Could you check a few things on this model? Use its own coordinates, in mm. Face numbers are marked on the shaded views. A direction names the side the tool comes from. Round coordinates to 2 decimals unless told otherwise and drop trailing zeros. Loops run counter-clockwise (first coordinate to the right, second up) from the corner with the lowest first, then second, coordinate; pieces in that order, holes last.
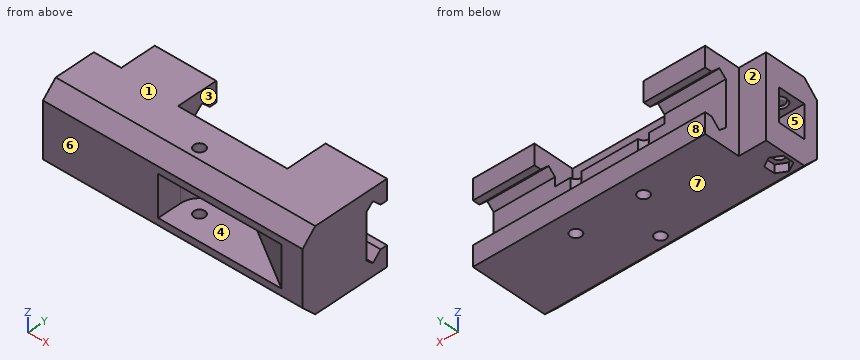
from build123d import *

# Parameters (mm, degrees)
SKETCH_1_W               = 30
SKETCH_1_H               = 20
SKETCH_1_W_2             = 12
SKETCH_1_H_2             = 10
EXTRUDE_1_DEPTH          = 10
CUT_EXTRUDE_1_DEPTH      = 3
SKETCH_4_R               = 1.95
CUT_EXTRUDE_2_DEPTH      = 30
SKETCH_8_R               = 2.8
SKETCH_8_R_2             = 2.2
CUT_EXTRUDE_3_DEPTH      = 5
FILLET_1_R               = 1
SKETCH_12_W              = 85
SKETCH_12_H              = 33.2
EXTRUDE_3_DEPTH          = 15
CUT_EXTRUDE_4_DEPTH      = 100
CHAMFER_1_SIZE           = 5
CUT_EXTRUDE_5_DEPTH      = 99.935534567
CUT_EXTRUDE_5_DEPTH_BACK = 99.935534567
SKETCH_14_R              = 2
CUT_EXTRUDE_6_DEPTH      = 7.5
CUT_EXTRUDE_7_DEPTH      = 99.935534567
CUT_EXTRUDE_7_DEPTH_BACK = 99.935534567
SKETCH_16_R              = 2
SKETCH_17_W              = 40
SKETCH_17_H              = 15
CUT_EXTRUDE_8_DEPTH      = 10


with BuildPart() as part:
    # 스케치1 → 보스-돌출1 (new body)
    with BuildSketch(Plane(origin=(0, 0, 0), x_dir=(0, 0, -1), z_dir=(1, 0, 0))):
        Rectangle(SKETCH_1_W, SKETCH_1_H)
        Rectangle(SKETCH_1_W_2, SKETCH_1_H_2, mode=Mode.SUBTRACT)
    extrude(amount=EXTRUDE_1_DEPTH)

    # 스케치2 → 컷-돌출1 (cut)
    with BuildSketch(Plane(origin=(0, 0, -15), x_dir=(-1, 0, 0), z_dir=(0, 0, -1))):
        Polygon((-1.175, -2.006292185), (-1.175, 2.006292185), (-4.65, 4.012584371), (-8.125, 2.006292185), (-8.125, -2.006292185), (-4.65, -4.012584371), align=None)
    extrude(amount=-CUT_EXTRUDE_1_DEPTH, mode=Mode.SUBTRACT)

    # 스케치4 → 컷-돌출2 (cut)
    with BuildSketch(Plane.XY):
        with Locations(Location((4.65, 0, 0), (0, 0, 270))):
            Circle(SKETCH_4_R)
    extrude(amount=-CUT_EXTRUDE_2_DEPTH, mode=Mode.SUBTRACT)

    # 스케치8 → 컷-돌출3 (cut)
    with BuildSketch(Plane(origin=(0, 0, 6), x_dir=(-1, 0, 0), z_dir=(0, 0, -1))):
        with Locations(Location((-4.65, 0, 0), (0, 0, 90))):
            Circle(SKETCH_8_R)
        with Locations(Location((-4.65, 0, 0), (0, 0, 90))):
            Circle(SKETCH_8_R_2, mode=Mode.SUBTRACT)
    extrude(amount=-CUT_EXTRUDE_3_DEPTH, mode=Mode.SUBTRACT)

    # 필렛1
    fillet_1_edges = [part.edges().sort_by_distance(p)[0] for p in [
        (4.65, -2.2, 6),
    ]]
    fillet(fillet_1_edges, radius=FILLET_1_R)

    # 스케치12 → 보스-돌출3 (add, symmetric)
    with BuildSketch(Plane.XY):
        with Locations((52.5, 6.6)):
            Rectangle(SKETCH_12_W, SKETCH_12_H)
    extrude(amount=EXTRUDE_3_DEPTH, both=True)

    # 스케치13 → 컷-돌출4 (cut, symmetric)
    with BuildSketch(Plane(origin=(0, 0, 0), x_dir=(0, 0, -1), z_dir=(1, 0, 0))):
        Polygon((7.6, 23.2), (-7.6, 23.2), (-7.6, 20.7), (-10.5, 17.7), (-10.5, 17.6), (-8.25, 15.1), (8.25, 15.1), (10.5, 17.6), (10.5, 17.7), (7.6, 20.7), align=None)
    extrude(amount=CUT_EXTRUDE_4_DEPTH, both=True, mode=Mode.SUBTRACT)

    # 모따기1
    chamfer_1_edges = [part.edges().sort_by_distance(p)[0] for p in [
        (47.5, -10, -15),
        (47.5, -10, 15),
    ]]
    chamfer(chamfer_1_edges, length=CHAMFER_1_SIZE)

    # 스케치14 → 컷-돌출5 (cut, two sides: drawn at the far end of the back side and taken through both)
    with BuildSketch(Plane.XY.offset(-CUT_EXTRUDE_5_DEPTH_BACK)):
        with Locations(Location((40.1, 15.1, 0), (0, 0, 90))):
            Circle(SKETCH_14_R)
        with Locations(Location((64.9, 15.1, 0), (0, 0, 90))):
            Circle(SKETCH_14_R)
    extrude(amount=CUT_EXTRUDE_5_DEPTH + CUT_EXTRUDE_5_DEPTH_BACK, mode=Mode.SUBTRACT)

    # 스케치15 → 컷-돌출6 (cut, symmetric)
    with BuildSketch(Plane.XY):
        with BuildLine():
            Line((62.713186115, 5.72501597), (49.092705045, 5.72501597))
            ThreePointArc((49.092705045, 5.72501597), (44.199467341, 3.698170549), (42.17262192, -1.195067155))
            Line((42.17262192, -1.195067155), (42.17262192, -12.628733774))
            Line((42.17262192, -12.628733774), (87.317926114, -12.628733774))
            Line((87.317926114, -12.628733774), (87.317926114, -10))
            Line((87.317926114, -10), (62.713186115, 5.72501597))
        make_face()
    extrude(amount=CUT_EXTRUDE_6_DEPTH, both=True, mode=Mode.SUBTRACT)

    # 스케치16 → 컷-돌출7 (cut, two sides: drawn at the far end of the back side and taken through both)
    with BuildSketch(Plane.XY.offset(-CUT_EXTRUDE_7_DEPTH_BACK)):
        with Locations((49.092705045, -1.195067155)):
            Circle(SKETCH_16_R)
    extrude(amount=CUT_EXTRUDE_7_DEPTH + CUT_EXTRUDE_7_DEPTH_BACK, mode=Mode.SUBTRACT)

    # 스케치17 → 컷-돌출8 (cut)
    with BuildSketch(Plane.XY.offset(15)):
        with Locations((52.5, 15.7)):
            Rectangle(SKETCH_17_W, SKETCH_17_H)
    extrude(amount=-CUT_EXTRUDE_8_DEPTH, mode=Mode.SUBTRACT)


solid = part.part
Item 1: We'd pull the mould along Y, two halves only. Please class the marked faces 5, 6, 7 and 8: released by +Y, released by -Y, zero draft, split by the parting line, or undercut.
Results list:
face 5: undercut
face 6: released by -Y
face 7: zero draft
face 8: released by +Y
Item 2: If we section it at D-D, the plane z = 3.5: Please give me the cut outline in (x, y).
Results list:
outline: (0, -10) - (42.17, -10) - (42.17, -1.2) arc R6.92 cw to (49.09, 5.73) - (62.71, 5.73) - (87.32, -10) - (95, -10) - (95, 15.1) - (66.9, 15.1) arc R2 cw to (62.9, 15.1) - (42.1, 15.1) arc R2 cw to (38.1, 15.1) - (10, 15.1) - (10, 10) - (0, 10) - (0, 5) - (10, 5) - (10, -5) - (0, -5) - close
Item 3: If we section it at B-B, the plane y = 11.5: Please give me the cut outline in (x, z), then the cut area to 3 significant figures.
Results list:
outline: (10, -15) - (95, -15) - (95, 15) - (72.5, 15) - (72.5, 5) - (32.5, 5) - (32.5, 15) - (10, 15) - close
area: 2,150 mm2
Item 4: If we section it at C-C, the plane x = 19.5: Please give me the cut outline in (y, z).
Results list:
outline: (-10, -10) - (-5, -15) - (23.2, -15) - (23.2, -7.6) - (20.7, -7.6) - (17.7, -10.5) - (17.6, -10.5) - (15.1, -8.25) - (15.1, 8.25) - (17.6, 10.5) - (17.7, 10.5) - (20.7, 7.6) - (23.2, 7.6) - (23.2, 15) - (-5, 15) - (-10, 10) - close
Item 5: If we section it at A-A, the plane x = 40.1: Please give me the cut outline in (y, z).
Results list:
outline: (-10, -10) - (-5, -15) - (13.1, -15) - (13.1, 5) - (8.2, 5) - (8.2, 15) - (-5, 15) - (-10, 10) - close; (17.1, -15) - (23.2, -15) - (23.2, -7.6) - (20.7, -7.6) - (17.7, -10.5) - (17.6, -10.5) - (17.1, -10.05) - close
Item 6: If I drill on line 1 along X through (y, z) = (15.1, -9); line 2 along Z through (x, y) = (62, 2); line 3 along X through (y, z) = (-0.5, -9), over which ranges is the centre line in solid material (lowest first)?
Results list:
line 1: x = 10 to 38.1, 42.1 to 62.9, 66.9 to 95
line 2: z = -15 to -7.5, 7.5 to 15
line 3: x = 0 to 2.77, 6.53 to 47.22, 50.97 to 95
Item 7: For the marked faces 1, 2, 3 and 4, which set-ups out of +Z, -Z, +X, -X, +Y, -Y let a thin tool reach every point of the face, with its end or its side?
Results list:
face 1: +Z, +X, -X, +Y, -Y
face 2: +Z, -Z, -X, +Y
face 3: +Z, +Y
face 4: -Y
Item 8: Will these pins go through, and if not, where does the flat tip stop? pin 1 (3 mm diameter, centred on x = 3.5, y = -0.5, fed in from -Z); pin 2 (3 mm diameter, centred on x = 54.5, z = 10, fed in from +Y); pin 3 (4 mm diameter, centred on y = -2.5, z = -11.5, fed in from -X); pin 4 (1 mm diameter, centred on x = 29, z = 4, fed in from +Y).
Results list:
pin 1: stops at z = -12
pin 2: stops at y = 8.2
pin 3: stops at x = 0
pin 4: stops at y = 15.1
